Read the model definition and answer for the solid it produces. Units are mm, in the model's axes. A direction names the side the tool comes from. Coordinates: 2 decimals unless noted, no trailing zeros. Order: outer loops, then holes, each group sorted by start corner. A loop starts at its lowest first (then second) coordinate and runs counter-clockwise, first axis right, second up.
```python
from build123d import *

# Parameters (mm, degrees)
BOSS_EXTRUDE1_START     = -6.3
BOSS_EXTRUDE1_DEPTH     = 8.35
CUT_EXTRUDE1_REACH      = 18.833
CUT_EXTRUDE1_END_RADIUS = 1.85
CIRPATTERN3_COUNT       = 4
SKETCH10_W              = 0.084438725
SKETCH10_H              = 2.05


with BuildPart() as part:
    # Sketch1 → Revolve1 (revolve)
    with BuildSketch(Plane.XY, mode=Mode.PRIVATE) as revolve1_sk:
        Polygon((-3.15, 0), (-1.85, 0.75055535), (-1.85, 5.347868077), (-0.85, 5.347868077), (-0.85, 14.95), (-2, 14.28604719), (-2, 6.21), (-3.15, 6.21), align=None)
    revolve(revolve1_sk.sketch.rotate(Axis((0, 0, 0), (0, 1, 0)), 270), axis=Axis((0, 0, 0), (0, 1, 0)))

    # Sketch3 → Boss-Extrude1 (add)
    with BuildSketch(Plane(origin=(0, 6.21, 0), x_dir=(1, 0, 0), z_dir=(0, 1, 0)).offset(BOSS_EXTRUDE1_START)):
        with BuildLine():
            Line((-0.575, -3.915561275), (0.575, -3.915561275))
            Line((0.575, -3.915561275), (0.575, -1.915561275))
            ThreePointArc((0.575, -1.915561275), (0, -2), (-0.575, -1.915561275))
            Line((-0.575, -1.915561275), (-0.575, -3.915561275))
        make_face()
    boss_extrude1 = extrude(amount=BOSS_EXTRUDE1_DEPTH)

    # Cut-Extrude1: up to this cylinder (the profile starts outside it)
    cut_extrude1_end = Plane(origin=(0, 7.980101, 0), z_dir=(0, -1, 0)) * Cylinder(CUT_EXTRUDE1_END_RADIUS, 42.366, mode=Mode.PRIVATE)
    # Sketch4 → Cut-Extrude1 (cut, up to the surface)
    with BuildSketch(Plane.XY.offset(3.915561275), mode=Mode.PRIVATE) as cut_extrude1_sk1:
        Polygon((0.575, 7.420304493), (-0.575, 8.26), (0.575, 8.26), align=None)
    cut_extrude1_tool1 = extrude(cut_extrude1_sk1.sketch, amount=-CUT_EXTRUDE1_REACH, mode=Mode.PRIVATE) - cut_extrude1_end
    cut_extrude1 = cut_extrude1_tool1.solids().sort_by_distance((0.191667, 7.980101, 3.915561))[0]
    add(cut_extrude1, mode=Mode.SUBTRACT)

    # CirPattern3: Boss-Extrude1, Cut-Extrude1 ×4 about axis
    cirpattern3_axis = Axis((0, 0, 0), (0, 1, 0))
    add([boss_extrude1.rotate(cirpattern3_axis, i * 360 / CIRPATTERN3_COUNT) for i in range(1, CIRPATTERN3_COUNT)])
    add([cut_extrude1.rotate(cirpattern3_axis, i * 360 / CIRPATTERN3_COUNT) for i in range(1, CIRPATTERN3_COUNT)], mode=Mode.SUBTRACT)

    # Sketch9 → Cut-Revolve2 (revolve, cut)
    with BuildSketch(Plane.XY, mode=Mode.PRIVATE) as cut_revolve2_sk:
        Polygon((-3.915561275, -0.09), (-1.85, 0.75055535), (-1.85, -0.09), align=None)
    revolve(cut_revolve2_sk.sketch.rotate(Axis((0, 0, 0), (0, -1, 0)), 90), axis=Axis((0, 0, 0), (0, -1, 0)), mode=Mode.SUBTRACT)

    # Sketch10 → Revolve2 (revolve)
    with BuildSketch(Plane.XY, mode=Mode.PRIVATE) as revolve2_sk:
        with Locations((-1.957780637, 7.235)):
            Rectangle(SKETCH10_W, SKETCH10_H)
    revolve(revolve2_sk.sketch.rotate(Axis((0, 0, 0), (0, -1, 0)), 90), axis=Axis((0, 0, 0), (0, -1, 0)))


solid = part.part
```
1) Which of the six approach directions +Z, -Z, +X, -X, +Y, -Y give full straight-line access (tool end or side, diameter ignored) to faces 1 (the flat face through (3.4, 3.6, -0.575)), 2 (the flat face through (0.575, 3.6, 3.4)), 3 (the flat face through (-2, 6.21, -2))?
A:
face 1: -Z, +X, +Y
face 2: +Z, +X, +Y
face 3: -Z, -X, +Y
2) Flat-ended cylindrical pins translate along their axes: pin 1 Ø1.6 at (x, y) = (-3, 3) entering from -Z; pin 2 Ø2 at (x, y) = (3, 5) entering from -Z; pin 3 Ø1.6 at (x, y) = (2.5, 2.5) entering from +Z; pin 4 Ø4 at (x, y) = (2, 6) entering from -Z. Find the tip coordinate at first contact, or state that the pin passes through.
A:
pin 1: stops at z = -2.25
pin 2: stops at z = -2.43
pin 3: stops at z = 2.65
pin 4: stops at z = -3.92
3) A cutting plane is placed at A-A, the plane y = 11.5. Determine the outline of the cut face in (x, z).
A:
outline: circle Ø4 at (0, 0); hole circle Ø1.7 at (0, 0)
4) Straight lines are drawn through the part: line 1 (X direction, y = 2.7, z = 0); line 2 (X direction, y = 9.5, z = 0); line 3 (Z direction, x = 3.5, y = 6.75) (3 decimals). For each, find the intervals that lie inside material, in ascending order.
A:
line 1: x = -3.92 to -1.85, 1.85 to 3.92
line 2: x = -2 to -0.85, 0.85 to 2
line 3: z = -0.575 to 0.575
